Input: dimensioned drawing with shaded views. Units: mm. Origin: part minimum x, y, z. Give positions to 0.01 mm unless a question says otherwise; leave off trailing zeros. Loops run counter-clockwise (first coordinate to the right, second up) from the corner with the lowest first, then second, coordinate; pieces in that order, holes last.
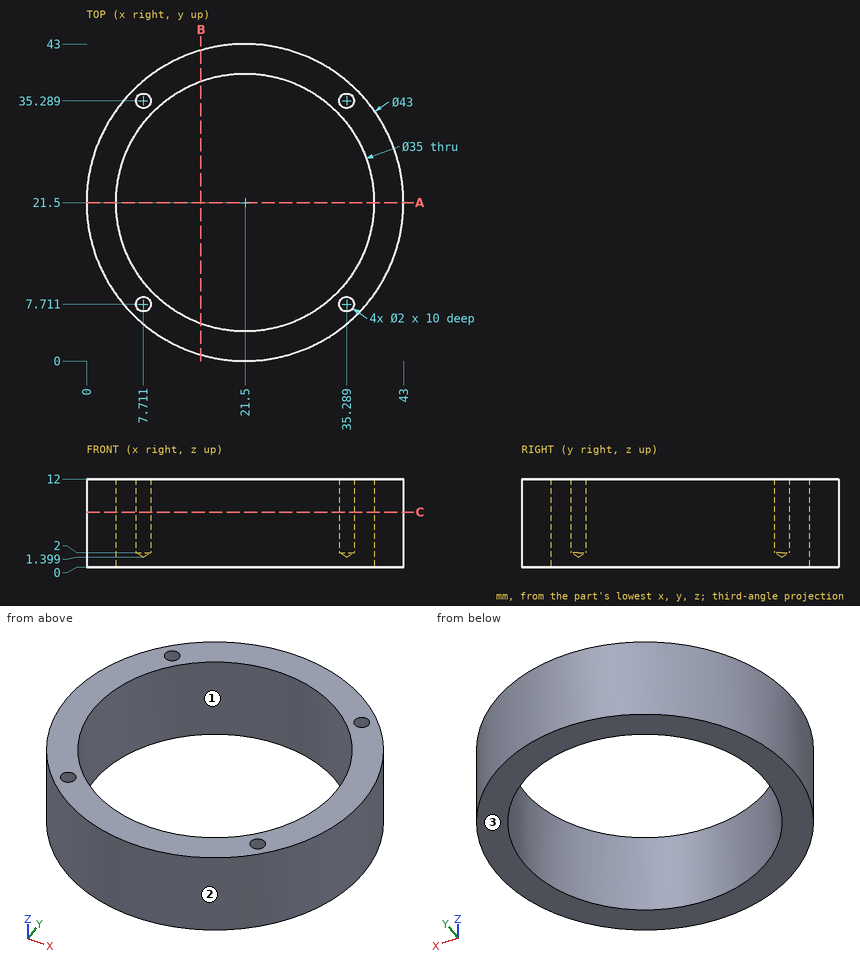
(1) Section C-C, the plane z = 7.5. Return the cut outline in (x, y).
A:
outline: circle Ø43 at (21.5, 21.5); hole circle Ø35 at (21.5, 21.5); hole circle Ø2 at (7.71, 7.71); hole circle Ø2 at (7.71, 35.29); hole circle Ø2 at (35.29, 7.71); hole circle Ø2 at (35.29, 35.29)
(2) Mould query, pull axis Y, two halves, no side actions, for the marked faces 1, 2 and 3. Classes: pulls with the +Y half, pulls with the -Y half, needs draft (parallel to the pull), parting line crosses it, or undercut.
A:
face 1: undercut
face 2: parting line crosses it
face 3: needs draft
(3) Ray query, line 1 along X through (y, z) = (35.5, 9.5) (1 decimal); line 2 along Y through (x, z) = (8, 5.5) (1 decimal); line 3 along Y through (x, z) = (21, 11.25) (1 decimal). Return the intervals inside material, ascending.
A:
line 1: x = 5.2 to 6.7, 8.7 to 11, 32 to 34.3, 36.3 to 37.8
line 2: y = 4.8 to 6.8, 8.7 to 10.4, 32.6 to 34.3, 36.2 to 38.2
line 3: y = 0 to 4, 39 to 43
(4) Section B-B, the plane x = 15.5. Return the cut outline in (y, z) (1 decimal), then the cut area to 3 significant figures.
A:
outline: (0.9, 0) - (5.1, 0) - (5.1, 12) - (0.9, 12) - close; (37.9, 0) - (42.1, 0) - (42.1, 12) - (37.9, 12) - close
area: 101 mm2
(5) Section A-A, the plane y = 21.5. Return the cut outline in (x, z).
A:
outline: (0, 0) - (4, 0) - (4, 12) - (0, 12) - close; (39, 0) - (43, 0) - (43, 12) - (39, 12) - close
(6) First-contact query: pin 1 (1 mm diameter, centred on x = 16, z = 5.5, fed in from +Y); pin 2 (6 mm diameter, centred on y = 32, z = 9.5, fed in from -X); pin 3 (2 mm diameter, centred on y = 9.5, z = 3, fed in from -X). Flat tips, straight axial feed; report the tip coordinate or a pass-through.
A:
pin 1: stops at y = 42.41
pin 2: stops at x = 1.35
pin 3: stops at x = 3.03
